Geometry: final body of the model. Coordinates: model frame, mm. Face numbers are marked on the shaded views. A direction names the side the tool comes from. Give positions to 0.01 mm unless a question says otherwise; leave off trailing zeros. Loops run counter-clockwise (first coordinate to the right, second up) from the corner with the lowest first, then second, coordinate; pieces in that order, holes last. Notation, with made-up numbers: (22, 78) -> (79, 78) arc R20 cw to (79, 117) -> close; hole circle Ø4 at (87.5, 39). An arc over 180 degrees is marked (long way). One line per question, with ' | ' between items. Start each with the question number.
Item 1: Section A-A on y = 17.5. Return loops of the section in (x, z).
Item 2: Section B-B on x = -15.9. Return loops of the section in (y, z).
Item 3: Pin query (flat end, axial travel): P1, Ø2, axis at y = 24.5, z = 8, coming from the +X side; P2, Ø7, axis at x = -15.9, z = 7, coming from the +Y side; P3, Ø6, axis at x = 16.5, z = 6, coming from the +Y side; P4, Ø3.5, axis at y = 24.09, z = 7, coming from the -X side. Return the tip coordinate at first contact, or that it passes through.
Item 4: Mould query, pull axis Y, two halves, no side actions, for the marked faces 1, 2, 3 and 4. Classes: released by +Y, released by -Y, zero draft, split by the parting line, or undercut.
Item 5: Set-up query: the marked faces 5, 6 and 7. Return all of +Z, -Z, +X, -X, +Y, -Y with unobstructed straight access to the full face (end or side cutting, diameter ignored); none if empty.
Item 6: Section C-C on z = 11.25. Return loops of the section in (x, y).
Item 7: Material intervals for line 1 along X through (y, z) = (-0.35, 7); line 2 along Y through (x, z) = (6.35, 7); line 3 along Y through (x, z) = (2.05, 7), sorted ascending. Write a range as [from, to].
Item 8: Section D-D on x = 7.5. Return loops of the section in (y, z), then the cut area to 3 significant figures.
from build123d import *

# Parameters (mm, degrees)
SKETCH1_R           = 4
BOSS_EXTRUDE1_DEPTH = 14
SKETCH2_R           = 2.75
CUT_EXTRUDE1_DEPTH  = 6
SKETCH3_W           = 2
SKETCH3_H           = 11.620769134
CUT_EXTRUDE2_DEPTH  = 14
SKETCH4_R           = 2
CUT_EXTRUDE3_DEPTH  = 9
SKETCH5_R           = 3.5
CUT_EXTRUDE4_DEPTH  = 4
SKETCH6_R           = 1.85
CUT_EXTRUDE5_DEPTH  = 9
FILLET1_R           = 0.3


with BuildPart() as part:
    # Sketch1 → Boss-Extrude1 (new body)
    with BuildSketch(Plane.XY):
        Polygon((-20.938905162, 0.786403392), (-9.238905162, 0.786403392), (-9.238905162, 28.586403392), (8.761094838, 28.586403392), (8.761094838, 1.886403392), (20.761094838, 1.886403392), (20.761094838, -4.713596608), (-20.938905162, -4.713596608), align=None)
        with Locations((0, 15.086403392)):
            Circle(SKETCH1_R, mode=Mode.SUBTRACT)
    extrude(amount=BOSS_EXTRUDE1_DEPTH)

    # Sketch2 → Cut-Extrude1 (cut)
    with BuildSketch(Plane(origin=(0, 1.886403392, 0), x_dir=(1, 0, 0), z_dir=(0, 1, 0))):
        with Locations((-15.9, -7)):
            Circle(SKETCH2_R)
        with Locations((15.9, -7)):
            Circle(SKETCH2_R)
    extrude(amount=-CUT_EXTRUDE1_DEPTH, mode=Mode.SUBTRACT)

    # Sketch3 → Cut-Extrude2 (cut)
    with BuildSketch(Plane.XY.offset(14)):
        with Locations((0.152630001, 23.872597077)):
            Rectangle(SKETCH3_W, SKETCH3_H)
    extrude(amount=-CUT_EXTRUDE2_DEPTH, mode=Mode.SUBTRACT)

    # Sketch4 → Cut-Extrude3 (cut)
    with BuildSketch(Plane(origin=(8.761094838, 0, 0), x_dir=(0, 0, -1), z_dir=(1, 0, 0))):
        with Locations((-7, 24.086403392)):
            Circle(SKETCH4_R)
    extrude(amount=-CUT_EXTRUDE3_DEPTH, mode=Mode.SUBTRACT)

    # Sketch5 → Cut-Extrude4 (cut)
    with BuildSketch(Plane(origin=(8.761094838, 0, 0), x_dir=(0, 0, -1), z_dir=(1, 0, 0))):
        with Locations((-7, 24.086403392)):
            Circle(SKETCH5_R)
    extrude(amount=-CUT_EXTRUDE4_DEPTH, mode=Mode.SUBTRACT)

    # Sketch6 → Cut-Extrude5 (cut)
    with BuildSketch(Plane.ZY.offset(9.238905162)):
        with Locations((7, 24.086403392)):
            Circle(SKETCH6_R)
    extrude(amount=-CUT_EXTRUDE5_DEPTH, mode=Mode.SUBTRACT)

    # Fillet1
    fillet1_edges = [part.edges().sort_by_distance(p)[0] for p in [
        (-20.938905162, 0.786403392, 7),
        (-9.238905162, 28.586403392, 7),
        (8.761094838, 28.586403392, 7),
        (20.761094838, 1.886403392, 7),
    ]]
    fillet(fillet1_edges, radius=FILLET1_R)


solid = part.part
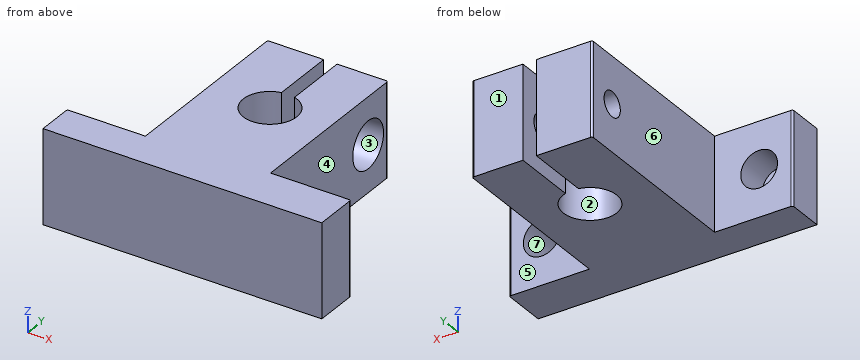
Result sheet:
1) outline: (-9.24, 0) -> (-3.19, 0) -> (-3.19, 14) -> (-9.24, 14) -> close; (3.19, 0) -> (8.76, 0) -> (8.76, 14) -> (3.19, 14) -> close
2) outline: (-4.71, 0) -> (0.79, 0) -> (0.79, 4.25) -> (-4.11, 4.25) -> (-4.11, 9.75) -> (0.79, 9.75) -> (0.79, 14) -> (-4.71, 14) -> close
3) P1: stops at x = 4.76 | P2: stops at y = 0.79 | P3: stops at y = 1.89 | P4: passes through
4) face 1: released by +Y | face 2: undercut | face 3: undercut | face 4: zero draft
5) face 5: +Z, -Z, +X, +Y | face 6: +Z, -Z, -X, +Y | face 7: +Y
6) outline: (-20.94, -4.71) -> (20.76, -4.71) -> (20.76, 1.59) arc R0.3 ccw to (20.46, 1.89) -> (8.76, 1.89) -> (8.76, 28.29) arc R0.3 ccw to (8.46, 28.59) -> (1.15, 28.59) -> (1.15, 18.92) arc R4 cw (long way) to (-0.85, 19) -> (-0.85, 28.59) -> (-8.94, 28.59) arc R0.3 ccw to (-9.24, 28.29) -> (-9.24, 0.79) -> (-20.64, 0.79) arc R0.3 ccw to (-20.94, 0.49) -> close
7) line 1: x = [-20.94, -18.65], [-13.15, 13.15], [18.65, 20.76] | line 2: y = [-4.71, 20.59], [27.59, 28.59] | line 3: y = [-4.71, 11.65], [18.52, 22.09], [26.09, 28.59]
8) outline: (-4.71, 0) -> (28.59, 0) -> (28.59, 14) -> (-4.71, 14) -> close; hole circle Ø7 at (24.09, 7) | area: 428 mm²
